Read the model definition and answer for the solid it produces. Units are mm, in the model's axes. A direction names the side the tool comes from. Round coordinates to 2 decimals unless told otherwise and drop trailing zeros. Write each loop counter-clockwise with the first axis right and the second up, starting at its lowest first coordinate (ties: lowest second). Pieces come first, ordered by that corner, then holes. Notation, with made-up numbers: (26, -20.5) -> (34, -20.5) arc R21 cw to (34, -3.5) -> close; hole circle Ø2 at (41.5, 9). An arc over 180 degrees is marked (long way). Return JSON: item names as keys, results as strings.
from build123d import *

# Parameters (mm, degrees)
SKETCH_1_W                  = 20
SKETCH_1_H                  = 20
EXTRUDE_1_DEPTH             = 20
SKETCH_2_W                  = 17
SKETCH_2_H                  = 17
CUT_EXTRUDE_1_DEPTH         = 66.429351212
HOLE_WIZARD_4_2_4_2_1_D     = 4.2
HOLE_WIZARD_4_2_4_2_1_DEPTH = 20
HOLE_WIZARD_4_0_4_1_D       = 4


with BuildPart() as part:
    # 草图1 → 凸台-拉伸1 (new body)
    with BuildSketch(Plane(origin=(0, 160, 0), x_dir=(1, 0, 0), z_dir=(0, 1, 0))):
        with Locations((49, -10)):
            Rectangle(SKETCH_1_W, SKETCH_1_H)
    extrude(amount=-EXTRUDE_1_DEPTH)

    # 草图2 → 切除-拉伸1 (cut, through all)
    with BuildSketch(Plane.XZ.offset(-140)):
        with Locations((50.5, 8.5)):
            Rectangle(SKETCH_2_W, SKETCH_2_H)
    extrude(amount=-CUT_EXTRUDE_1_DEPTH, mode=Mode.SUBTRACT)

    # Ø4.2 (4.2) 直径孔1
    with Locations(Plane.ZY.offset(-39)):
        with Locations((10, 150)):
            Hole(HOLE_WIZARD_4_2_4_2_1_D / 2, depth=HOLE_WIZARD_4_2_4_2_1_DEPTH)

    # Ø4.0 (4) 直径孔1 (through all)
    with Locations(Plane(origin=(0, 0, 17), x_dir=(-1, 0, 0), z_dir=(0, 0, -1))):
        with Locations((-49, 145), (-49, 155)):
            Hole(HOLE_WIZARD_4_0_4_1_D / 2)


solid = part.part
Item 1: Flat-ended cylindrical pins translate along their axes: pin 1 (10 mm diameter, centred on x = 46.5, y = 157.5, fed in from -Z); pin 2 (2 mm diameter, centred on y = 145, z = 2.5, fed in from +X); pin 3 (4.5 mm diameter, centred on x = 49, y = 155, fed in from -Z); pin 4 (2.5 mm diameter, centred on x = 49, y = 145, fed in from -Z). Find the tip coordinate at first contact, or state that the pin passes through.
Worked answers:
{"pin 1": "stops at z = 0", "pin 2": "stops at x = 42", "pin 3": "stops at z = 17", "pin 4": "passes through"}
Item 2: A tool of negligible diameter and unlimited length cuts with its end or side. For faces 5 (the flat face through (40, 150, 0)), 6 (the flat face through (50, 150, 17)), from which of +Z, -Z, +X, -X, +Y, -Y can it reach the whole face along a straight path? Write none if from no direction.
Worked answers:
{"face 5": "-Z, +X, -X, +Y, -Y", "face 6": "-Z, +X, +Y, -Y"}
Item 3: Section D-D (y = 141.75) is taken. Give the vertices of the cut face in (x, z).
Worked answers:
{"outline": "(39, 0) -> (42, 0) -> (42, 17) -> (59, 17) -> (59, 20) -> (39, 20) -> close"}
Item 4: Section A-A (y = 145) is taken. Give the vertices of the cut face in (x, z), then the cut area to 3 significant figures.
Worked answers:
{"outline": "(39, 0) -> (42, 0) -> (42, 17) -> (47, 17) -> (47, 20) -> (39, 20) -> close; (51, 17) -> (59, 17) -> (59, 20) -> (51, 20) -> close", "area": "99.0 mm2"}
Item 5: Section B-B (x = 49) is taken. Give the vertices of the cut face in (y, z), then the cut area to 3 significant figures.
Worked answers:
{"outline": "(140, 17) -> (143, 17) -> (143, 20) -> (140, 20) -> close; (147, 17) -> (153, 17) -> (153, 20) -> (147, 20) -> close; (157, 17) -> (160, 17) -> (160, 20) -> (157, 20) -> close", "area": "36.0 mm2"}
Item 6: For a pull along X with two mould halves and no side action, classify faces 1 (the flat face through (39, 152.4, 10.1)), 2 (the flat face through (41.5, 160, 13.7)), 3 (the cylindrical face through (49.923, 153.226, 18.521)), 4 (the flat face through (59, 150, 19)) as released by +X, released by -X, zero draft, split by the parting line, or undercut.
Worked answers:
{"face 1": "released by -X", "face 2": "zero draft", "face 3": "undercut", "face 4": "released by +X"}
Item 7: Straight lines are drawn through the part: L1, parallel to Y at x = 49, z = 17.6; L2, parallel to Z at x = 40.05, y = 150; L3, parallel to Y at x = 39.9, z = 10. For each, find the intervals that lie inside material, in ascending order. Write a range as [from, to].
Worked answers:
{"L1": "y = [140, 143], [147, 153], [157, 160]", "L2": "z = [0, 7.9], [12.1, 20]", "L3": "y = [140, 147.9], [152.1, 160]"}
Item 8: Section C-C (z = 11) is taken. Give the vertices of the cut face in (x, y).
Worked answers:
{"outline": "(39, 140) -> (42, 140) -> (42, 148.15) -> (39, 148.15) -> close; (39, 151.85) -> (42, 151.85) -> (42, 160) -> (39, 160) -> close"}
